```python
from build123d import *

# Parameters (mm, degrees)
SKETCH_1_W          = 28.9
SKETCH_1_H          = 20
SKETCH_1_R          = 1.65
EXTRUDE_1_DEPTH     = 5
SKETCH_1_5_W        = 28.9
SKETCH_1_5_H        = 5
EXTRUDE_4_DEPTH     = 25
SKETCH_2_W          = 25
SKETCH_2_H          = 20
SKETCH_2_R          = 1.75
EXTRUDE_5_DEPTH     = 5
SKETCH_3_W          = 28.9
SKETCH_3_H          = 20
SKETCH_3_R          = 1.65
EXTRUDE_6_DEPTH     = 4.5
CUT_EXTRUDE_1_REACH = 61.418
SKETCH_4_R          = 3.5


with BuildPart() as part:
    # Sketch 1 → Extrude 1 (new body)
    with BuildSketch(Plane.XY):
        with Locations((14.45, 10)):
            Rectangle(SKETCH_1_W, SKETCH_1_H)
        with Locations((9.45, 17.5)):
            Circle(SKETCH_1_R, mode=Mode.SUBTRACT)
        with Locations((19.45, 17.5)):
            Circle(SKETCH_1_R, mode=Mode.SUBTRACT)
        with Locations((9.45, 2.5)):
            Circle(SKETCH_1_R, mode=Mode.SUBTRACT)
        with Locations((19.45, 2.5)):
            Circle(SKETCH_1_R, mode=Mode.SUBTRACT)
    extrude(amount=EXTRUDE_1_DEPTH)

    # Sketch 1_5 → Extrude 4 (add)
    with BuildSketch(Plane.XY):
        with Locations((14.45, -2.5)):
            Rectangle(SKETCH_1_5_W, SKETCH_1_5_H)
        with Locations((14.45, 22.5)):
            Rectangle(SKETCH_1_5_W, SKETCH_1_5_H)
    extrude(amount=EXTRUDE_4_DEPTH)

    # Sketch 2 → Extrude 5 (add)
    with BuildSketch(Plane(origin=(28.9, 0, 0), x_dir=(0, 0, -1), z_dir=(1, 0, 0))):
        with Locations((12.5, 10)):
            Rectangle(SKETCH_2_W, SKETCH_2_H)
        with Locations(Location((20, 10, 0), (0, 0, 90))):
            Circle(SKETCH_2_R, mode=Mode.SUBTRACT)
        with Locations(Location((6, 10, 0), (0, 0, 90))):
            Circle(SKETCH_2_R, mode=Mode.SUBTRACT)
    extrude(amount=-EXTRUDE_5_DEPTH)

    # Sketch 3 → Extrude 6 (add)
    with BuildSketch(Plane.XY.offset(25)):
        with Locations((14.45, 10)):
            Rectangle(SKETCH_3_W, SKETCH_3_H)
        with Locations((14.45, 10)):
            Circle(SKETCH_3_R, mode=Mode.SUBTRACT)
    extrude(amount=-EXTRUDE_6_DEPTH)

    # Sketch 4 → Cut-Extrude 1 (cut, up to next)
    with BuildSketch(Plane(origin=(0, 0, 20.5), x_dir=(-1, 0, 0), z_dir=(0, 0, -1)), mode=Mode.PRIVATE) as cut_extrude_1_sk1:
        with Locations(Location((-14.45, 10, 0), (0, 0, 180))):
            Circle(SKETCH_4_R)
    cut_extrude_1_tool1 = extrude(cut_extrude_1_sk1.sketch, amount=CUT_EXTRUDE_1_REACH, mode=Mode.PRIVATE) & part.part
    add(cut_extrude_1_tool1.solids().sort_by_distance((14.45, 10, 20.5))[0], mode=Mode.SUBTRACT)


solid = part.part
```
Design review of the part built by this model. Coordinates are the model's own, in mm. A direction names the side the tool comes from. Coordinates: 2 decimals unless noted, no trailing zeros. Loops run counter-clockwise (first coordinate to the right, second up) from the corner with the lowest first, then second, coordinate; pieces in that order, holes last. Notation, with made-up numbers: (39, 3.25) - (74, 3.25) arc R20 ccw to (74, 8.25) - close; hole circle Ø4 at (74, -23.5). An arc over 180 degrees is marked (long way). Use CSV: the item, a comma, the result in double quotes. Start each with the question number.
1) The part is to be moulded in two halves that separate along Z. For faces 1 (the flat face through (14, 20, 13)), 2 (the flat face through (26, 20, -12)), 3 (the flat face through (11, 10, 25)), say which applies: +Z half, -Z half, draft (parallel to the pull), parting line (faces both ways), or undercut.
2) Wall thickness on L1, parallel to Z at x = 26.7, y = 10; L2, parallel to Y at x = 19.45, z = 1.1; L3, parallel to Z at x = 5, y = 15.75: over which ranges is each line inside the solid? List them lowest first. Write a range as from..to.
3) Consider section C-C on y = 2.5. Write out the cut boundary in (x, z), then the cut area to 3 significant figures.
4) Consider section B-B on x = 22.5. Write out the cut boundary in (y, z), then the cut area to 3 significant figures.
5) Consider section D-D on z = 4. Write out the cut boundary in (x, y), then the cut area to 3 significant figures.
6) Tool access review of faces 4 (the cylindrical face through (18.234, 18.615, 2.465)), 5 (the flat face through (23.9, 10, -12)), 6 (the flat face through (14, 8, 20.5)), 7 (the flat face through (28.9, 10, 0)), 8 (the flat face through (26, 0, -12)): name each direction out of +Z, -Z, +X, -X, +Y, -Y from which nothing blocks a thin tool from reaching the whole face with its end or side.
7) Consider section A-A on x = 14.45. Write out the cut boundary in (y, z).
8) For pin 1 Ø5.5 at (x, y) = (19.45, 17.5) entering from -Z; pin 2 Ø10 at (y, z) = (13, -18) entering from -X; pin 3 Ø2.5 at (x, z) = (25.5, -16) entering from +Y, all flat-tipped, find the tip position at first contact; note any pin that passes through.
Geometry says:
1,face 1,"undercut"
1,face 2,"draft"
1,face 3,"+Z half"
2,L1,"-25..-21.75, -18.25..-7.75, -4.25..5, 20.5..25"
2,L2,"-5..0.85, 4.15..15.85, 19.15..25"
2,L3,"0..5, 20.5..25"
3,outline,"(0, 0) - (7.8, 0) - (7.8, 5) - (0, 5) - close; (0, 20.5) - (28.9, 20.5) - (28.9, 25) - (0, 25) - close; (11.1, 0) - (17.8, 0) - (17.8, 5) - (11.1, 5) - close; (21.1, 0) - (23.9, 0) - (23.9, -25) - (28.9, -25) - (28.9, 5) - (21.1, 5) - close"
3,area,"367 mm^2"
4,outline,"(-5, 0) - (25, 0) - (25, 25) - (-5, 25) - close; hole (0, 5) - (20, 5) - (20, 20.5) - (0, 20.5) - close"
4,area,"440 mm^2"
5,outline,"(0, -5) - (28.9, -5) - (28.9, 25) - (0, 25) - close; hole circle Ø3.3 at (9.45, 2.5); hole circle Ø3.3 at (9.45, 17.5); hole circle Ø7 at (14.45, 10); hole circle Ø3.3 at (19.45, 2.5); hole circle Ø3.3 at (19.45, 17.5)"
5,area,"794 mm^2"
6,face 4,"-Z"
6,face 5,"-Z, -X, +Y, -Y"
6,face 6,"+X, -X"
6,face 7,"+Z, -Z, +X, +Y, -Y"
6,face 8,"-Z, +X, -X, -Y"
7,outline,"(-5, 0) - (6.5, 0) - (6.5, 5) - (0, 5) - (0, 20.5) - (8.35, 20.5) - (8.35, 25) - (-5, 25) - close; (11.65, 20.5) - (20, 20.5) - (20, 5) - (13.5, 5) - (13.5, 0) - (25, 0) - (25, 25) - (11.65, 25) - close"
8,pin 1,"z = 0"
8,pin 2,"x = 23.9"
8,pin 3,"y = 20"
